Verification items for this drawing (mm, ordinates from the low corner). A direction names the side the tool comes from. Give positions to 0.01 mm unless a question says otherwise; leave off trailing zeros. Loops run counter-clockwise (first coordinate to the right, second up) from the corner with the lowest first, then second, coordinate; pieces in that order, holes last. Notation, with made-up numbers: (75, 80) -> (111, 80) arc R16 ccw to (111, 94) -> close; hole circle Ø11 at (69, -20.5). An arc over 180 degrees is marked (long way). Write item = value, one per line.
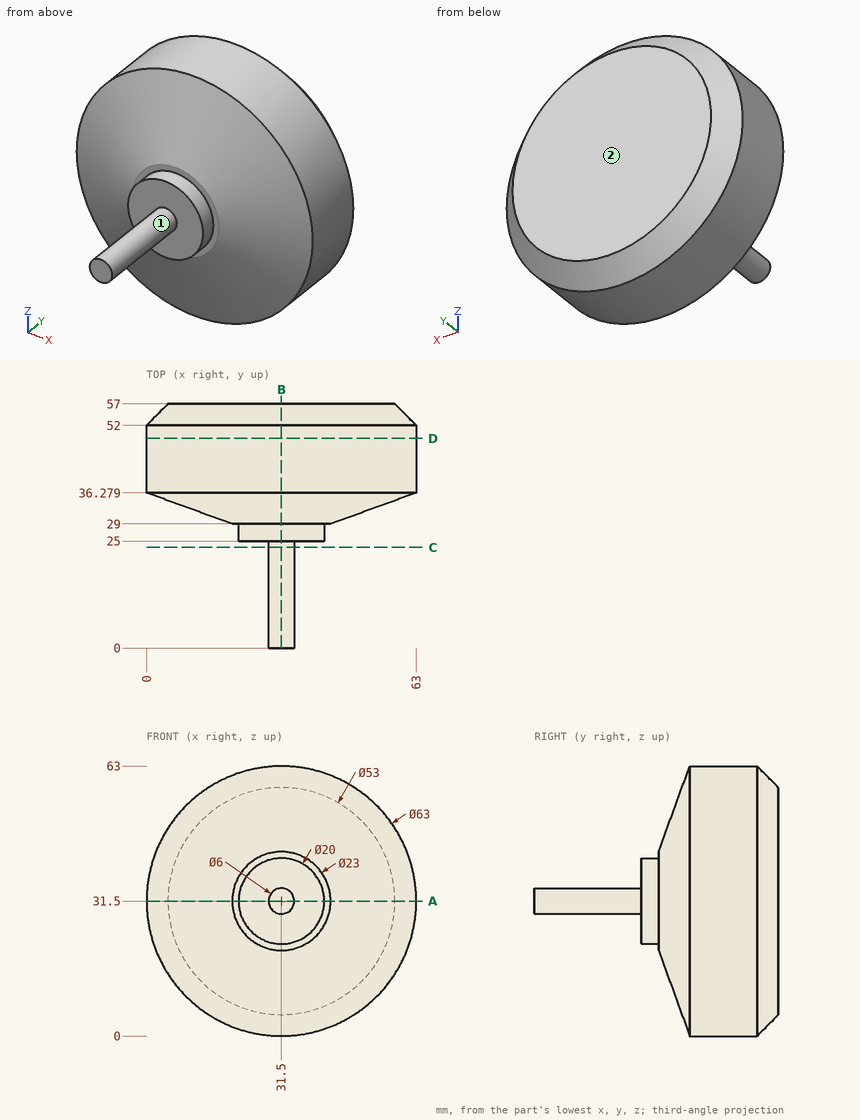
Item 1: Section check C-C, the plane y = 23.5. Record the cut outline in (x, z).
Answer:
outline = circle Ø6 at (31.5, 31.5)
Item 2: Section check D-D, the plane y = 49. Record the cut outline in (x, z), plus the area to 3 significant figures.
Answer:
outline = circle Ø63 at (31.5, 31.5)
area = 3,120 mm^2
Item 3: Section check B-B, the plane x = 31.5. Record the cut outline in (y, z), plus the area to 3 significant figures.
Answer:
outline = (0, 28.5) -> (25, 28.5) -> (25, 21.5) -> (29, 21.5) -> (29, 20) -> (36.28, 0) -> (52, 0) -> (57, 5) -> (57, 58) -> (52, 63) -> (36.28, 63) -> (29, 43) -> (29, 41.5) -> (25, 41.5) -> (25, 34.5) -> (0, 34.5) -> close
area = 1,820 mm^2
Item 4: Thickness scan on L1, parallel to X at y = 48, z = 32; L2, parallel to Y at x = 45, z = 48.5 (1 decimal); L3, parallel to Y at x = 50, z = 37. Record the ranges inside material, lowest first. Write a range as [from, to].
Answer:
L1 = [0, 63]
L2 = [32.7, 57]
L3 = [31.84, 57]
Item 5: Section check A-A, the plane z = 31.5. Record the cut outline in (x, y), plus the area to 3 significant figures.
Answer:
outline = (0, 36.28) -> (20, 29) -> (21.5, 29) -> (21.5, 25) -> (28.5, 25) -> (28.5, 0) -> (34.5, 0) -> (34.5, 25) -> (41.5, 25) -> (41.5, 29) -> (43, 29) -> (63, 36.28) -> (63, 52) -> (58, 57) -> (5, 57) -> (0, 52) -> close
area = 1,820 mm^2
Item 6: Tool access check on the marked faces 1 and 2. Record the directions out of +Z, -Z, +X, -X, +Y, -Y that give a thin tool (end or side, any length) a straight path to the whole face; none if there is none.
Answer:
face_1 = -Y
face_2 = +Z, -Z, +X, -X, +Y
Item 7: Gauge pin test, flat ends, axial feed: pin 1 (1.5 mm diameter, centred on x = 27, z = 9, fed in from -Y); pin 2 (2 mm diameter, centred on x = 49, z = 25.5, fed in from -Y); pin 3 (1.5 mm diameter, centred on y = 27.5, z = 21.5, fed in from -X). Record the tip position at first contact, or that the pin passes through.
Answer:
pin_1 = 32.89
pin_2 = 31.18
pin_3 = 27.7
